```python
from build123d import *

# Parameters (mm, degrees)
F0_R     = 9
F1_DEPTH = 40
F3_DEPTH = 80
F5_DEPTH = 100
F7_R     = 10
F8_DEPTH = 100


with BuildPart() as f1:
    # F0 (on Front) → F1 (new body)
    with BuildSketch(Plane.XZ):
        with BuildLine():
            ThreePointArc((-20, 0), (0, -20), (20, 0))
            ThreePointArc((20, 0), (14.1421356237, 14.1421356237), (0, 20))
            ThreePointArc((0, 20), (-14.1421356237, 14.1421356237), (-20, 0))
        make_face()
        Circle(F0_R, mode=Mode.SUBTRACT)
        with BuildLine():
            Line((20, -10), (20, 0))
            ThreePointArc((20, 0), (0, -20), (-20, 0))
            Line((-20, 0), (-20, -10))
            ThreePointArc((-20, -10), (-22.9289321881, -17.0710678119), (-30, -20))
            Line((-30, -20), (-40, -20))
            Line((-40, -20), (-40, -60))
            Line((-40, -60), (40, -60))
            Line((40, -60), (40, -20))
            Line((40, -20), (30, -20))
            ThreePointArc((30, -20), (22.9289321881, -17.0710678119), (20, -10))
        make_face()
    extrude(amount=F1_DEPTH)

    # F2 (on face) → F3 (join)
    with BuildSketch(Plane(origin=(-40, 0, 0), x_dir=(0, -1, 0), z_dir=(-1, 0, 0))):
        Polygon((-18, -60), (0, -60), (0, -20), (0, 20), (-68, 20), (-68, -50), (-28, -50), align=None)
    extrude(amount=-F3_DEPTH)


with BuildPart() as f5:
    # F4 (on face) → F5 (new body)
    with BuildSketch(Plane.XY.offset(20)):
        Polygon((20, 68), (-20, 68), (-25, 56), (0, 56), (25, 56), align=None)
    extrude(amount=-F5_DEPTH)


with BuildPart() as f1_1:
    add(f1.part)

    # F6: cut F5
    add(f5.part, mode=Mode.SUBTRACT)


with BuildPart() as f8:
    # F7 (on face) → F8 (new body)
    with BuildSketch(Plane.XY.offset(20)):
        with Locations((0, 28)):
            Circle(F7_R)
    extrude(amount=-F8_DEPTH)


with BuildPart() as f1_2:
    add(f1_1.part)

    # F9: cut F8
    add(f8.part, mode=Mode.SUBTRACT)


solid = f1_2.part
```
Could you check a few things on this model? Use its own coordinates, in mm. A direction names the side the tool comes from. Coordinates: 2 decimals unless noted, no trailing zeros. Write each loop counter-clockwise with the first axis right and the second up, starting at its lowest first coordinate (ties: lowest second). Pieces come first, ordered by that corner, then holes. Notation, with made-up numbers: (79.5, 56.25) -> (122.5, 56.25) arc R33 ccw to (122.5, 84.25) -> close; hole circle Ø7 at (-29, 16). An arc over 180 degrees is marked (long way). Write item = value, one per line. Start each with the question number.
(1) I want a section at D-D (x = 6.5). Please give me the cut outline in (y, z), plus the area to 3 significant figures.
(2) We'd pull the mould along X, two halves only. Please class faces 1 (the face through (-22.465, 62.084, -14.51)), 2 (the face through (-22.85, -19.72, -16.99)), 3 (the face through (30, 68, -15)): released by +X, released by -X, zero draft, split by the parting line, or undercut.
(3) Will these pins go through, and if not, where does the flat tip stop? pin 1 (5 mm diameter, centred on y = -20, z = -4, fed in from +X); pin 2 (3 mm diameter, centred on x = 1, y = 57, fed in from -Z); pin 3 (9 mm diameter, centred on x = -1.5, z = -2.5, fed in from -Y).
(4) I need wall thicknesses on line 1 (Y direction, x = 0, z = -12); line 2 (Y direction, x = 0, z = -1); line 3 (Z direction, x = 27.5, y = 43). Which ranges of each line are inside material? Lowest first, please. Write a range as [from, to].
(5) I want a section at C-C (y = 22.5). Please give me the cut outline in (x, z), plus the area to 3 significant figures.
(6) I want a section at A-A (y = -19.5). Please give me the cut outline in (x, z).
(7) Which directions (+Z, -Z, +X, -X, +Y, -Y) give clear straight access to the entire face, cutting with the end or side of a thin tool? Please do faces 4 (the face through (-1, 48, -50)), 5 (the face through (0, 0, 0)), 6 (the face through (22.535, 61.916, -14.51)), 7 (the face through (-35, -20, -20)), 8 (the face through (23.01, -19.72, -17.15)).
(8) I want a section at B-B (z = -18). Please give me the cut outline in (x, y), plus the area to 3 significant figures.
Result set:
q1.outline = (-40, -60) -> (18, -60) -> (20.4, -57.6) -> (20.4, 20) -> (0, 20) -> (0, 18.91) -> (-40, 18.91) -> (-40, 6.22) -> (0, 6.22) -> (0, -6.22) -> (-40, -6.22) -> close; (35.6, -50) -> (56, -50) -> (56, 20) -> (35.6, 20) -> close
q1.area = 5,720 mm2
q2.face_1 = undercut
q2.face_2 = released by -X
q2.face_3 = zero draft
q3.pin_1 = 20
q3.pin_2 = -50
q3.pin_3 = 0
q4.line_1 = [-40, 18], [38, 56]
q4.line_2 = [0, 18], [38, 56]
q4.line_3 = [-50, 20]
q5.outline = (-40, -55.5) -> (-8.35, -55.5) -> (-8.35, 20) -> (-40, 20) -> close; (8.35, -55.5) -> (40, -55.5) -> (40, 20) -> (8.35, 20) -> close
q5.area = 4,780 mm2
q6.outline = (-40, -60) -> (40, -60) -> (40, -20) -> (30, -20) arc R10 cw to (20, -10) -> (20, 0) arc R20 ccw to (-20, 0) -> (-20, -10) arc R10 cw to (-30, -20) -> (-40, -20) -> close; hole circle Ø18 at (0, 0)
q7.face_4 = -Z, +X, -X, +Y
q7.face_5 = -Y
q7.face_6 = +Z, -Z
q7.face_7 = +Z, -X, -Y
q7.face_8 = +Z, +X, -Y
q8.outline = (-40, 0) -> (-24, 0) -> (-24, -40) -> (24, -40) -> (24, 0) -> (40, 0) -> (40, 68) -> (20, 68) -> (25, 56) -> (-25, 56) -> (-20, 68) -> (-40, 68) -> close; hole circle Ø20 at (0, 28)
q8.area = 6,510 mm2
